Build history of the part. All positions in model axes, mm. Coordinates: 2 decimals unless noted, no trailing zeros. Order: outer loops, then holes, each group sorted by start corner. A loop starts at its lowest first (then second) coordinate and runs counter-clockwise, first axis right, second up. Notation, with made-up numbers: (75.5, 44) -> (79.5, 44) arc R25 cw to (79.5, 64) -> close; hole circle Ø8 at (18, -33). An arc over 180 degrees is marked (long way). Write each question's results on one line, items separated by ' | '.
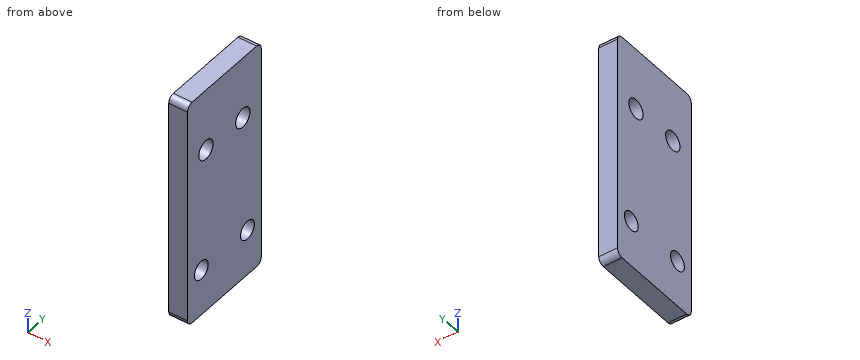
from build123d import *

# Parameters (mm, degrees)
SKETCH_1_W      = 37
SKETCH_1_H      = 16
SKETCH_1_R      = 1.5
SKETCH_1_R_2    = 1.55
EXTRUDE_1_DEPTH = 3
FILLET_1_R      = 1


with BuildPart() as part:
    # 草图1 → 凸台-拉伸1 (new body)
    with BuildSketch(Plane(origin=(0, 0, 0), x_dir=(0, 0, -1), z_dir=(1, 0, 0))):
        Rectangle(SKETCH_1_W, SKETCH_1_H)
        with Locations((11, 5)):
            Circle(SKETCH_1_R, mode=Mode.SUBTRACT)
        with Locations((11, -5)):
            Circle(SKETCH_1_R, mode=Mode.SUBTRACT)
        with Locations((-8.5, 4)):
            Circle(SKETCH_1_R_2, mode=Mode.SUBTRACT)
        with Locations((-8.5, -4)):
            Circle(SKETCH_1_R_2, mode=Mode.SUBTRACT)
    extrude(amount=EXTRUDE_1_DEPTH)

    # 圆角1
    fillet_1_edges = [part.edges().sort_by_distance(p)[0] for p in [
        (1.5, 8, 18.5),
        (1.5, 8, -18.5),
        (1.5, -8, -18.5),
        (1.5, -8, 18.5),
    ]]
    fillet(fillet_1_edges, radius=FILLET_1_R)


solid = part.part
Item 1: Drill centre lines: line 1 (Y direction, x = 1.65, z = -11); line 2 (Y direction, x = 0.6, z = 8.5); line 3 (Z direction, x = 2.05, y = -4.5). Where is each one in solid material? Low to high. Write a range as from..to.
Answer:
line 1: y = -8..-6.5, -3.5..3.5, 6.5..8 | line 2: y = -8..-5.55, -2.45..2.45, 5.55..8 | line 3: z = -18.5..-12.41, -9.59..7.03, 9.97..18.5
Item 2: Slice it at C-C, the plane y = -4. List the corners of the cut face in (x, z), and give its area (3 significant figures).
Answer:
outline: (0, -18.5) -> (3, -18.5) -> (3, -12.12) -> (0, -12.12) -> close; (0, -9.88) -> (3, -9.88) -> (3, 6.95) -> (0, 6.95) -> close; (0, 10.05) -> (3, 10.05) -> (3, 18.5) -> (0, 18.5) -> close | area: 95.0 mm^2
Item 3: Slice it at A-A, the plane z = 8.5. List the corners of the cut face in (x, y), and give its area (3 significant figures).
Answer:
outline: (0, -8) -> (3, -8) -> (3, -5.55) -> (0, -5.55) -> close; (0, -2.45) -> (3, -2.45) -> (3, 2.45) -> (0, 2.45) -> close; (0, 5.55) -> (3, 5.55) -> (3, 8) -> (0, 8) -> close | area: 29.4 mm^2
Item 4: Slice it at B-B, the plane x = 1.25. List the corners of the cut face in (y, z), and give its area (3 significant figures).
Answer:
outline: (-8, -17.5) arc R1 ccw to (-7, -18.5) -> (7, -18.5) arc R1 ccw to (8, -17.5) -> (8, 17.5) arc R1 ccw to (7, 18.5) -> (-7, 18.5) arc R1 ccw to (-8, 17.5) -> close; hole circle Ø3 at (-5, -11); hole circle Ø3.1 at (-4, 8.5); hole circle Ø3.1 at (4, 8.5); hole circle Ø3 at (5, -11) | area: 562 mm^2
